Autodesk Inventor part; units mm, degrees
ref_plane "XZ Plane" through (0, 0, 0) normal (0, 1, 0) x (-1, 0, 0)
ref_plane "XY Plane" through (0, 0, 0) normal (0, 0, 1) x (1, 0, 0)
sketch "Эскиз1" plane through (0, 0, 0) normal (0, 0, 1) x (1, 0, 0)
  line L0 (-32.5, -7.5) -> (32.5, -7.5)
  line L1 (32.5, -7.5) -> (32.5, 7.5)
  line L2 (32.5, 7.5) -> (-32.5, 7.5)
  line L3 (-32.5, -7.5) -> (32.5, 7.5) construction
  line L4 (32.5, -7.5) -> (-32.5, 7.5) construction
  line L5 (-32.5, 7.5) -> (-47.5, 7.5)
  line L6 (-47.5, 7.5) -> (-47.5, -22.5)
  line L7 (-47.5, -22.5) -> (-32.5, -22.5)
  line L8 (-32.5, -22.5) -> (-32.5, -7.5)
  line L9 (-32.5, -7.5) -> (-32.5, 7.5)
  point P0 (0, 0)
  dimension "d5" = 65
  dimension "d6" = 15
  dimension "d7" = 30
  dimension "d8" = 15
extrude "Выдавливание1" add sketch "Эскиз1" along normal mid plane 57
sketch "Эскиз2" plane through (0, 0, 28.5) normal (0, 0, 1) x (1, 0, 0)
  circle A0 centre (-40, -17) radius 2
  circle A1 centre (23.5, 0) radius 2
  line L0 (-47.5, -22.5) -> (-32.5, -22.5)
  line L1 (-40, -22.5) -> (-40, 7.5) construction
  line L2 (32.5, 7.5) -> (-47.5, 7.5)
  line L3 (32.5, -7.5) -> (32.5, 7.5)
  circle A2 centre (23.5, 0) radius 2
  point P0 (0, 0)
  dimension "d9" = 4
  dimension "d10" = 5.5
  dimension "d17" = 9
extrude "Выдавливание2" cut sketch "Эскиз2" against normal up to surface (57 mm away)
fillet "Сопряжение1" radius 10 3 edges at (-47.5, 7.5, 0) (-47.5, -22.5, 0) (-32.5, -7.5, 0)
fillet "Сопряжение2" radius 5 1 edges at (-32.5, -22.5, 0)
fillet "Сопряжение4" radius 7.5 2 edges at (32.5, 7.5, 0) (32.5, -7.5, 0)
properties part number "Фиксатор головы"
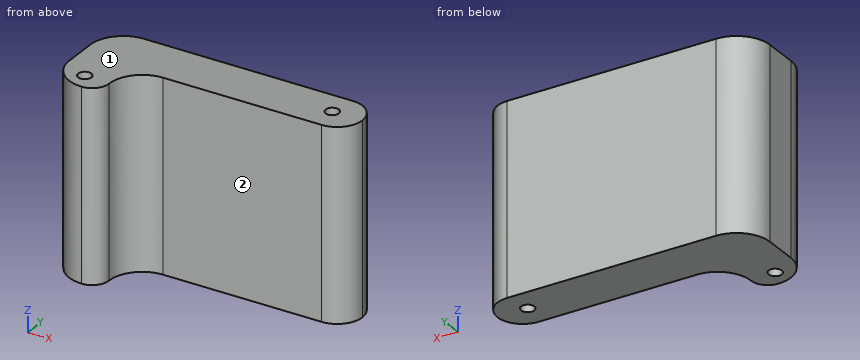
Here's how the part is built. I have some questions about the finished solid (model axes, mm). Face numbers are marked on the shaded views. A direction names the side the tool comes from. Round coordinates to 2 decimals unless told otherwise and drop trailing zeros. Loops run counter-clockwise (first coordinate to the right, second up) from the corner with the lowest first, then second, coordinate; pieces in that order, holes last. Notation, with made-up numbers: (1.5, 54) - (27.5, 54) arc R30 cw to (27.5, 84) - close; hole circle Ø4 at (4, 23.25). An arc over 180 degrees is marked (long way). One line per question, with ' | ' between items. Start each with the question number.
Q1. I want a section at C-C (x = -40). Write out the boundary of the cut face in (y, z), then the cut area to 3 significant figures.
Q2. For the marked faces 1 and 2, which set-ups out of +Z, -Z, +X, -X, +Y, -Y let a thin tool reach every point of the face, with its end or its side?
Q3. Will these pins go through, and if not, where does the flat tip stop? pin 1 (6 mm diameter, centred on y = -8.5, z = -14.5, fed in from +X); pin 2 (5 mm diameter, centred on y = -15.5, z = 10.5, fed in from +X).
Q4. I want a section at D-D (y = -5.5). Write out the boundary of the cut face in (x, z).
Q5. Please list where these lines run through material, in increasing order: line 1 (Y direction, x = 23.5, z = 2.5); line 2 (X direction, y = 1, z = 5); line 3 (Y direction, x = -1.5, z = -7). Write a range as [from, to].
Q6. I want a section at A-A (x = 23.5). Write out the boundary of the cut face in (y, z).
Q7. I want a section at B-B (z = -12.5). State how many separate pieces and enclosed holes the cut face has, then the cut area to 3 significant figures.
Response values:
1) outline: (-22.18, -28.5) - (-19, -28.5) - (-19, 28.5) - (-22.18, 28.5) - close; (-15, -28.5) - (7.18, -28.5) - (7.18, 28.5) - (-15, 28.5) - close | area: 1,450 mm²
2) face 1: +Z, +X, -X, +Y, -Y | face 2: +Z, -Z, +X, -Y
3) pin 1: stops at x = 30.1 | pin 2: stops at x = -31.43
4) outline: (-47.5, -28.5) - (30.1, -28.5) - (30.1, 28.5) - (-47.5, 28.5) - close
5) line 1: y = [-7.5, -2], [2, 7.5] | line 2: x = [-46.87, 21.77], [25.23, 32.43] | line 3: y = [-7.5, 7.5]
6) outline: (-7.5, -28.5) - (-2, -28.5) - (-2, 28.5) - (-7.5, 28.5) - close; (2, -28.5) - (7.5, -28.5) - (7.5, 28.5) - (2, 28.5) - close
7) separate pieces: 1 | enclosed holes: 2 | area: 1,350 mm²
